Build history of the part. All positions in model axes, mm. A direction names the side the tool comes from. Round coordinates to 2 decimals unless told otherwise and drop trailing zeros. Loops run counter-clockwise (first coordinate to the right, second up) from the corner with the lowest first, then second, coordinate; pieces in that order, holes last. Notation, with made-up numbers: (-24.5, 63.25) - (14.5, 63.25) arc R16 cw to (14.5, 67.25) - close; hole circle Ø4 at (-19.75, -17). An arc over 180 degrees is marked (long way). Use a Markdown table: item, result.
from build123d import *

# Parameters (mm, degrees)
F0_W        = 40
F0_H        = 75
F1_DEPTH    = 40
F3_D        = 10
F4_T1_DEPTH = 175
F5_T1_DEPTH = 175
F6_R        = 6
F8_DEPTH    = 75.0010001
F9_R        = 1


# Not quite as in the source:
# - a fillet or chamfer that OpenCascade refuses, or shapes differently, is made with other operations: its cross-section is extruded or revolved along the edge and cut away or added


with BuildPart() as f1:
    # F0 (on Top) → F1 (new body)
    with BuildSketch(Plane.XY):
        Rectangle(F0_W, F0_H)
    extrude(amount=F1_DEPTH)

    # F3 (through all)
    with Locations(Plane.XY.offset(40)):
        with Locations((0, 25), (0, -25)):
            Hole(F3_D / 2)

    # F4: fillet of radius 20 on 1 edges, made by hand

    # F4_s2 → F4_t1 (cut)
    with BuildSketch(Plane.XZ.offset(-87.5)):
        with BuildLine():
            ThreePointArc((20, 20), (14.1421356237, 34.1421356237), (0, 40))
            Line((0, 40), (20, 40))
            Line((20, 40), (20, 20))
        make_face()
    extrude(amount=F4_T1_DEPTH, mode=Mode.SUBTRACT)

    # F5: fillet of radius 20 on 1 edges, made by hand

    # F5_s2 → F5_t1 (cut)
    with BuildSketch(Plane.XZ.offset(-87.5)):
        with BuildLine():
            ThreePointArc((-20, 20), (-14.1421356237, 34.1421356237), (0, 40))
            Line((0, 40), (-20, 40))
            Line((-20, 40), (-20, 20))
        make_face()
    extrude(amount=F5_T1_DEPTH, mode=Mode.SUBTRACT)

    # F6
    f6_edges = [f1.edges().sort_by_distance(p)[0] for p in [
        (-20, 0, 0),
        (20, 0, 0),
    ]]
    fillet(f6_edges, radius=F6_R)

    # F7 (on face) → F8 (cut, through all)
    with BuildSketch(Plane.XZ.offset(37.5)):
        with BuildLine():
            Line((-16, 20), (-16, 4))
            Line((-16, 4), (16, 4))
            Line((16, 4), (16, 20))
            ThreePointArc((16, 20), (0, 36), (-16, 20))
        make_face()
    extrude(amount=-F8_DEPTH, mode=Mode.SUBTRACT)

    # F9
    f9_edges = [f1.edges().sort_by_distance(p)[0] for p in [
        (-16, 0, 4),
        (16, 0, 4),
    ]]
    fillet(f9_edges, radius=F9_R)


solid = f1.part
Q1. Pull direction X, two halves, no side cores. Call faces 3 (the face through (1.08, -29.88, 1.97)), 4 (the face through (18.196, 0.525, 1.711)), 5 (the face through (0, -1, 36)), 6 (the face through (-1.6, -37.5, 3.6)): pulls with the +X half, pulls with the -X half, needs draft (parallel to the pull), parting line crosses it, or undercut.
Results found:
| item | result |
|---|---|
| face 3 | undercut |
| face 4 | pulls with the +X half |
| face 5 | undercut |
| face 6 | needs draft |
Q2. Which spindle directions (+Z, -Z, +X, -X, +Y, -Y) get a long thin tool onto all of the face, cutting with end or side? Do faces 1 (the face through (-16, -1, 13)), 2 (the face through (-18.289, 0.525, 1.804)). Say none if no direction does.
Results found:
| item | result |
|---|---|
| face 1 | +Y, -Y |
| face 2 | -Z, -X, +Y, -Y |
Q3. Cut at D-D, the plane y = 24. List the corners of the cut face in (x, z).
Results found:
| item | result |
|---|---|
| outline | (-20, 6) arc R6 ccw to (-14, 0) - (-4.9, 0) - (-4.9, 4) - (-15, 4) arc R1 cw to (-16, 5) - (-16, 20) arc R16 cw to (-4.9, 35.23) - (-4.9, 39.39) arc R20 ccw to (-20, 20) - close; (4.9, 0) - (14, 0) arc R6 ccw to (20, 6) - (20, 20) arc R20 ccw to (4.9, 39.39) - (4.9, 35.23) arc R16 cw to (16, 20) - (16, 5) arc R1 cw to (15, 4) - (4.9, 4) - close |
Q4. Drop flat-ended pins along their axis: pin 1 (12 mm diameter, centred on x = -6, z = 33.5, fed in from -Y); pin 2 (6 mm diameter, centred on x = 0, y = 25, fed in from -Z); pin 3 (10 mm diameter, centred on x = -9, y = -13, fed in from +Z); pin 4 (2 mm diameter, centred on x = 12, y = 8, fed in from +Z). Give the stop position or say it passes through.
Results found:
| item | result |
|---|---|
| pin 1 | stops at y = -37.5 |
| pin 2 | passes through |
| pin 3 | stops at z = 39.6 |
| pin 4 | stops at z = 36.7 |
Q5. Cut at A-A, the plane x = 13. List the corners of the cut face in (y, z).
Results found:
| item | result |
|---|---|
| outline | (-37.5, 0) - (37.5, 0) - (37.5, 4) - (-37.5, 4) - close; (-37.5, 29.33) - (37.5, 29.33) - (37.5, 35.2) - (-37.5, 35.2) - close |
Q6. Cut at C-C, the plane z = 26.5. List the corners of the cut face in (x, y), plus the area to 3 significant figures.
Results found:
| item | result |
|---|---|
| outline | (-18.91, -37.5) - (-14.62, -37.5) - (-14.62, 37.5) - (-18.91, 37.5) - close; (14.62, -37.5) - (18.91, -37.5) - (18.91, 37.5) - (14.62, 37.5) - close |
| area | 644 mm2 |
Q7. Probe line 1 (Y direction, x = 0, z = 1.25); line 2 (X direction, y = -14.5, z = 20.5); line 3 (X direction, y = 0, z = 33). List the from-to ranges inside material, lowest first.
Results found:
| item | result |
|---|---|
| line 1 | y = -37.5 to -30, -20 to 20, 30 to 37.5 |
| line 2 | x = -19.99 to -15.99, 15.99 to 19.99 |
| line 3 | x = -15.2 to -9.33, 9.33 to 15.2 |
Q8. Cut at B-B, the plane y = 2. List the corners of the cut face in (x, z).
Results found:
| item | result |
|---|---|
| outline | (-20, 6) arc R6 ccw to (-14, 0) - (14, 0) arc R6 ccw to (20, 6) - (20, 20) arc R20 ccw to (-20, 20) - close; hole (-16, 5) arc R1 ccw to (-15, 4) - (15, 4) arc R1 ccw to (16, 5) - (16, 20) arc R16 ccw to (-16, 20) - close |
